from build123d import *

# Parameters (mm, degrees)
F1_DEPTH = 320
F2_R     = 1.5
F3_R     = 0.5
F4_R     = 2.5
F5_DEPTH = 1.501


with BuildPart() as f1:
    # F0 (on Right) → F1 (new body)
    with BuildSketch(Plane.YZ):
        Polygon((0, 1.5), (0, 0), (51.65659, 0), (51.65659, 255), (50.15659, 255), (50.15659, 1.5), align=None)
    extrude(amount=F1_DEPTH)

    # F2
    f2_edges = [f1.edges().sort_by_distance(p)[0] for p in [
        (160, 51.65659, 0),
    ]]
    fillet(f2_edges, radius=F2_R)

    # F3
    f3_edges = [f1.edges().sort_by_distance(p)[0] for p in [
        (160, 50.15659, 1.5),
    ]]
    fillet(f3_edges, radius=F3_R)

    # F4 (on face) → F5 (cut, through all)
    with BuildSketch(Plane.XY.offset(1.5)):
        with Locations((15, 35.15659)):
            Circle(F4_R)
        with Locations((15, 10)):
            Circle(F4_R)
        with Locations((160, 10)):
            Circle(F4_R)
        with Locations((160, 35.15659)):
            Circle(F4_R)
        with Locations((305, 35.15659)):
            Circle(F4_R)
        with Locations((305, 10)):
            Circle(F4_R)
    extrude(amount=-F5_DEPTH, mode=Mode.SUBTRACT)


solid = f1.part
Model file for the job. Use its own axes, mm. A direction names the side the tool comes from. Coordinates: 2 decimals unless noted, no trailing zeros. Loops run counter-clockwise (first coordinate to the right, second up) from the corner with the lowest first, then second, coordinate; pieces in that order, holes last. Notation, with made-up numbers: (64, -17) -> (71, -17) arc R19 cw to (71, 1) -> close; hole circle Ø8 at (9.5, 74). An arc over 180 degrees is marked (long way). Use one line per item in the form item = value. Start each with the question number.
(1) Cut at A-A on x = 52.5. Give the cut face in (y, z), and give its area (3 significant figures).
(2) Probe probe 1 along Y at (x, z) = (160, 0.4); probe 2 along Y at (x, z) = (15, 0.95); probe 3 along Y at (x, z) = (100, 150). List the from-to ranges inside material, lowest first. Write a range as from..to.
(3) Flat gauge pin, fed straight in: pin 1 (15 mm diameter, centred on x = 236, y = 20, fed in from +Z). Where does the tip first touch, or does it go through?
(4) Cut at C-C on z = 111.5. Give the cut face in (x, y).
(5) Cut at B-B on y = 26.5. Give the cut face in (x, z).
(6) Tool access for faces 1 (the flat face through (158, 25, 0)), 2 (the flat face through (158, 50.157, 130)): list every direction of +Z, -Z, +X, -X, +Y, -Y with a clear straight run to the whole face (end or side of a thin tool).
Values:
q1.outline = (0, 0) -> (50.16, 0) arc R1.5 ccw to (51.66, 1.5) -> (51.66, 255) -> (50.16, 255) -> (50.16, 2) arc R0.5 cw to (49.66, 1.5) -> (0, 1.5) -> close
q1.area = 457 mm2
q2.probe_1 = 0..7.5, 12.5..32.66, 37.66..51.18
q2.probe_2 = 0..7.5, 12.5..32.66, 37.66..51.55
q2.probe_3 = 50.16..51.66
q3.pin_1 = 1.5
q4.outline = (0, 50.16) -> (320, 50.16) -> (320, 51.66) -> (0, 51.66) -> close
q5.outline = (0, 0) -> (320, 0) -> (320, 1.5) -> (0, 1.5) -> close
q6.face_1 = -Z, +X, -X, +Y, -Y
q6.face_2 = +Z, +X, -X, -Y
